Read the model definition and answer for the solid it produces. Units are mm, in the model's axes. Coordinates: 2 decimals unless noted, no trailing zeros. Order: outer loops, then holes, each group sorted by start corner. A loop starts at its lowest first (then second) coordinate and runs counter-clockwise, first axis right, second up. Notation, with made-up numbers: M 17.5,84 L 61.5,84 A31 cw 61.5,112 Z; hole C 41.5,21.25 d3. An arc over 180 degrees is marked long. Write each question's results on one line, items separated by ' | '.
```python
from build123d import *

# Parameters (mm, degrees)
F0_R     = 7.9375
F1_DEPTH = 13.716
F2_R     = 3.175
F3_SCALE = 1.4


with BuildPart() as f1:
    # F0 (on Top) → F1 (new body)
    with BuildSketch(Plane.XY):
        Polygon((6.8740766425, 11.90625), (-6.8740766425, 11.90625), (-13.7481532851, 0), (-6.8740766425, -11.90625), (6.8740766425, -11.90625), (13.7481532851, 0), align=None)
        Circle(F0_R, mode=Mode.SUBTRACT)
    extrude(amount=F1_DEPTH)

    # F2
    f2_edges = [f1.edges().sort_by_distance(p)[0] for p in [
        (-13.748153, 0, 6.858),
        (10.311115, -5.953125, 0),
        (13.748153, 0, 6.858),
        (6.874077, -11.90625, 6.858),
        (-6.874077, -11.90625, 6.858),
        (6.874077, 11.90625, 6.858),
        (-6.874077, 11.90625, 6.858),
        (0, -11.90625, 0),
        (-10.311115, -5.953125, 0),
        (-10.311115, 5.953125, 0),
        (0, 11.90625, 0),
        (10.311115, 5.953125, 0),
    ]]
    fillet(f2_edges, radius=F2_R)


with BuildPart() as f1_1:
    # F3: moved
    add(f1.part.scale(F3_SCALE))


solid = f1_1.part
```
(1) Given pin 1 (3 mm diameter, centred on x = -12, z = 7.5, fed in from +Y); pin 2 (10 mm diameter, centred on y = -11, z = 9.5, fed in from -X); pin 3 (4 mm diameter, centred on x = 14, z = 13.5, fed in from -Y); pin 4 (12 mm diameter, centred on x = -6.5, y = 3.5, fed in from -Z), each flat-ended and moving along its own axis, determine where each tip first touches the part or whether it passes through.
Conclusion:
pin 1: y = 15.04 | pin 2: x = -15.78 | pin 3: y = -12.55 | pin 4: z = 0
(2) The part is cut by section A-A, the plane x = 0. Write down the section's boundary in (y, z) (1 decimal).
Conclusion:
outline: M -16.7,4.4 A4.4 ccw -12.2,0 L -11.1,0 L -11.1,19.2 L -16.7,19.2 Z; M 11.1,0 L 12.2,0 A4.4 ccw 16.7,4.4 L 16.7,19.2 L 11.1,19.2 Z
(3) The mould has two halves that part along X. Classify faces 1 (the cylindrical face through (-0.099, 15.401, 1.337)), 2 (the flat face through (-14.485, -8.249, 11.72)), 3 (the cylindrical face through (13.29, 7.79, 1.34)), 4 (the cylindrical face through (5.974, 9.37, 9.467)): pulls with the +X half, pulls with the -X half, needs draft (parallel to the pull), parting line crosses it, or undercut.
Conclusion:
face 1: needs draft | face 2: pulls with the -X half | face 3: pulls with the +X half | face 4: undercut
(4) The part is cut by section C-C, the plane x = -6. Write down the section's boundary in (y, z) (3 decimals), then the cut area to 3 significant figures.
Conclusion:
outline: M -16.669,4.445 A4.445 ccw -12.224,0 L -9.353,0 L -9.353,19.202 L -16.669,19.202 Z; M 9.353,0 L 12.224,0 A4.445 ccw 16.669,4.445 L 16.669,19.202 L 9.353,19.202 Z | area: 272 mm²
(5) The part is cut by section D-D, the plane y = -15. Write down the section's boundary in (x, z) (3 decimals).
Conclusion:
outline: M -10.529,4.445 A3.471 ccw -7.057,0.974 L 7.057,0.974 A3.471 ccw 10.529,4.445 L 10.529,19.202 L -10.529,19.202 Z
(6) The part is cut by section B-B, the plane z = 16.25. Write down the section's boundary in (x, y) (1 decimal), then the cut area to 3 significant figures.
Conclusion:
outline: M -18,-2.2 L -10.9,-14.4 A4.4 ccw -7.1,-16.7 L 7.1,-16.7 A4.4 ccw 10.9,-14.4 L 18,-2.2 A4.4 ccw 18,2.2 L 10.9,14.4 A4.4 ccw 7.1,16.7 L -7.1,16.7 A4.4 ccw -10.9,14.4 L -18,2.2 A4.4 ccw Z; hole C 0,0 d22.2 | area: 568 mm²
(7) Straight lines are drawn through the part: line 1 (Y direction, x = 0, z = 13.5); line 2 (X direction, y = -10, z = 16.5); line 3 (Y direction, x = -10, z = 8). For each, find the intervals that lie inside material, in ascending order.
Conclusion:
line 1: -16.67 to -11.11, 11.11 to 16.67 | line 2: -13.47 to -4.85, 4.85 to 13.47 | line 3: -15.56 to -4.85, 4.85 to 15.56
